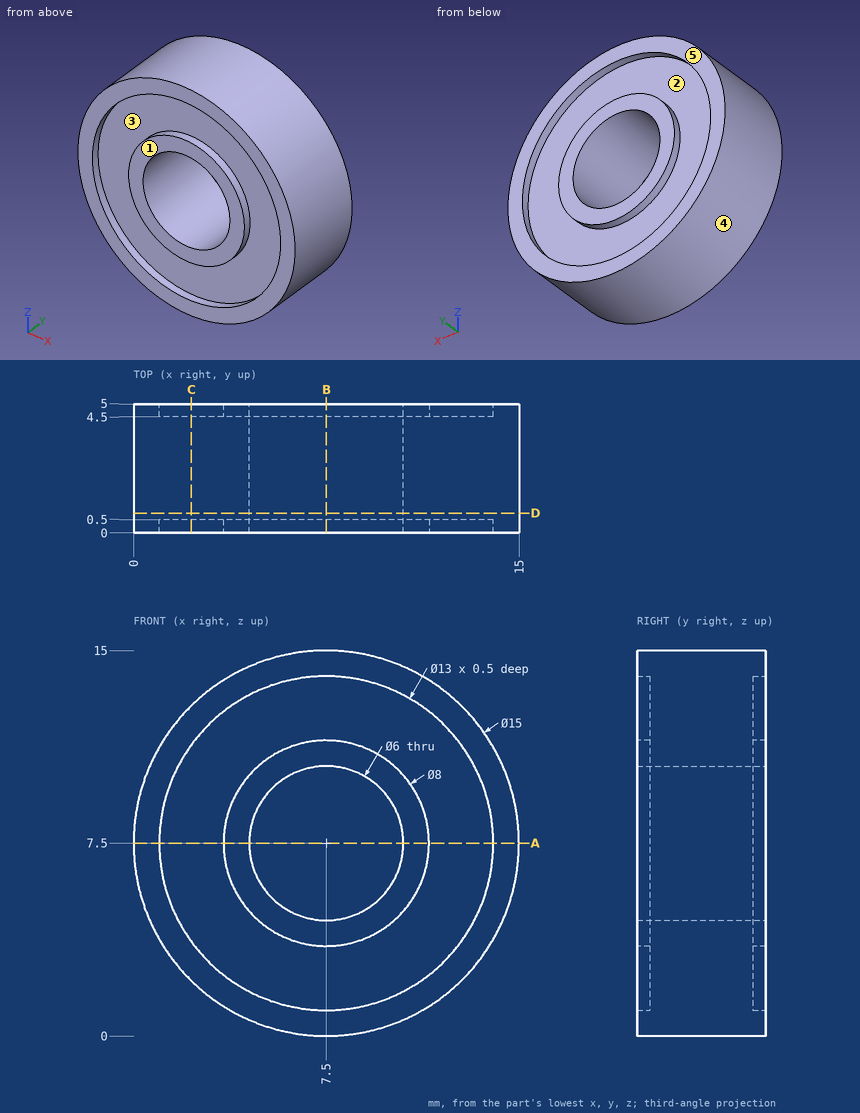
Design review of the part shown in the three views and the two pictorial views. Dimensions are in mm from the part's minimum x, y and z. A direction names the side the tool comes from. Round coordinates to 2 decimals unless told otherwise and drop trailing zeros. Loops run counter-clockwise (first coordinate to the right, second up) from the corner with the lowest first, then second, coordinate; pieces in that order, holes last. Notation, with made-up numbers: (-37.5, 14.25) - (6.5, 14.25) arc R12 cw to (6.5, 32.25) - close; hole circle Ø8 at (-5.5, 85.5). An arc over 180 degrees is marked (long way). Use one line per item in the form item = value.
1) Tool access review of the marked faces 1 and 2: name each direction out of +Z, -Z, +X, -X, +Y, -Y from which nothing blocks a thin tool from reaching the whole face with its end or side.
Solutions:
face_1 = +Z, -Z, +X, -X, -Y
face_2 = +Y
2) We need section C-C on x = 2.25. Write out the cut boundary in (y, z).
Solutions:
outline = (0, 2.14) - (5, 2.14) - (5, 3.67) - (4.5, 3.67) - (4.5, 11.33) - (5, 11.33) - (5, 12.86) - (0, 12.86) - (0, 11.33) - (0.5, 11.33) - (0.5, 3.67) - (0, 3.67) - close
3) Mouldability with a two-part tool opening along X and no side actions: class the marked faces 3, 4 and 5 as pulls with the +X half, pulls with the -X half, needs draft (parallel to the pull), parting line crosses it, or undercut.
Solutions:
face_3 = undercut
face_4 = parting line crosses it
face_5 = needs draft
4) We need section A-A on z = 7.5. Write out the cut boundary in (x, y), then the cut area to 3 significant figures.
Solutions:
outline = (0, 0) - (1, 0) - (1, 0.5) - (3.5, 0.5) - (3.5, 0) - (4.5, 0) - (4.5, 5) - (3.5, 5) - (3.5, 4.5) - (1, 4.5) - (1, 5) - (0, 5) - close; (10.5, 0) - (11.5, 0) - (11.5, 0.5) - (14, 0.5) - (14, 0) - (15, 0) - (15, 5) - (14, 5) - (14, 4.5) - (11.5, 4.5) - (11.5, 5) - (10.5, 5) - close
area = 40.0 mm2
5) We need section D-D on y = 0.75. Write out the cut boundary in (x, z), then the cut area to 3 significant figures.
Solutions:
outline = circle Ø15 at (7.5, 7.5); hole circle Ø6 at (7.5, 7.5)
area = 148 mm2
6) We need section B-B on x = 7.5. Write out the cut boundary in (y, z).
Solutions:
outline = (0, 0) - (5, 0) - (5, 1) - (4.5, 1) - (4.5, 3.5) - (5, 3.5) - (5, 4.5) - (0, 4.5) - (0, 3.5) - (0.5, 3.5) - (0.5, 1) - (0, 1) - close; (0, 10.5) - (5, 10.5) - (5, 11.5) - (4.5, 11.5) - (4.5, 14) - (5, 14) - (5, 15) - (0, 15) - (0, 14) - (0.5, 14) - (0.5, 11.5) - (0, 11.5) - close
7) Clearance check with flat-ended pins moving along their axes: P1, Ø3.5, axis at x = 7.5, z = 7.5, coming from the +Y side; P2, Ø2, axis at x = 4.5, y = 2, coming from the +Z side; P3, Ø1.5, axis at x = 4, y = 2.5, coming from the -Z side. State where each tip first meets the part, or that it passes through.
Solutions:
P1 = through
P2 = 14.73
P3 = 0.52
8) Wall thickness on probe 1 along Z at (x, y) = (7.5, 0.35); probe 2 along Z at (x, y) = (7.5, 2.1); probe 3 along X at (y, z) = (4.7, 7): over which ranges is each line inside the solid? List them lowest first.
Solutions:
probe_1 = 0 to 1, 3.5 to 4.5, 10.5 to 11.5, 14 to 15
probe_2 = 0 to 4.5, 10.5 to 15
probe_3 = 0.02 to 1.02, 3.53 to 4.54, 10.46 to 11.47, 13.98 to 14.98
